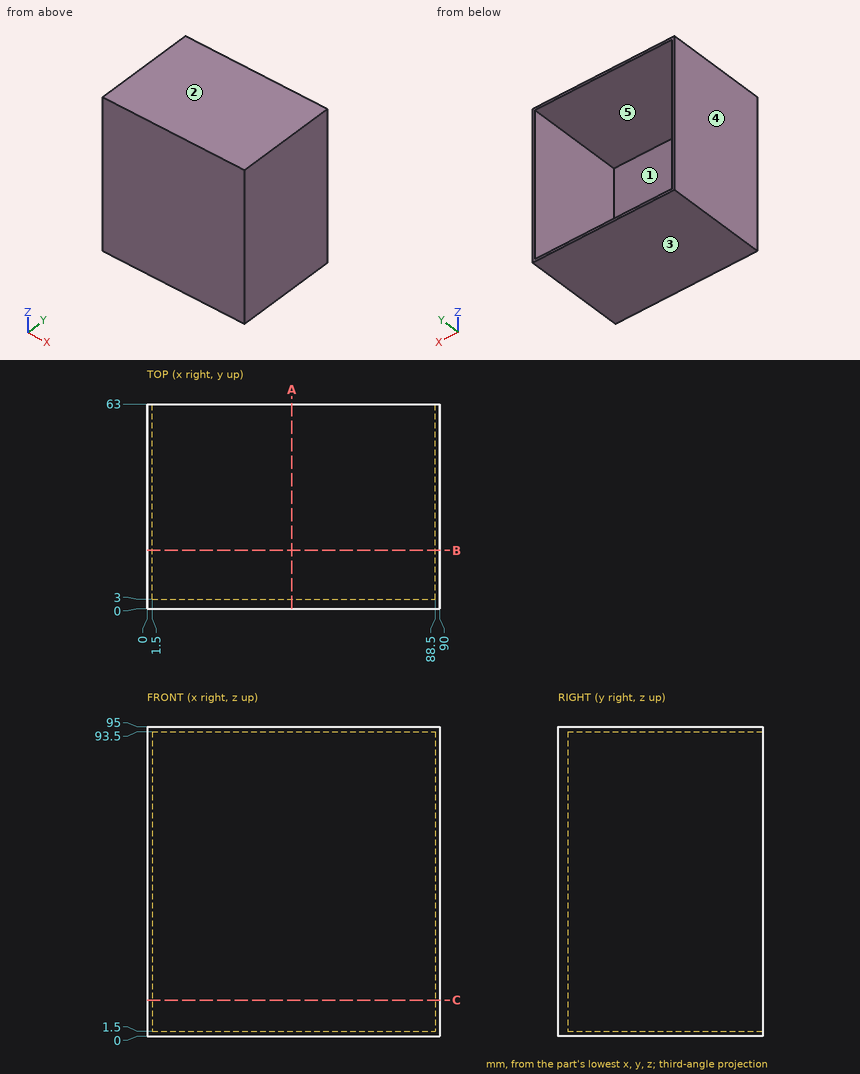
Check sheet for the drawn part. Datum: minimum x, y, z corner. Units: mm. A direction names the side the tool comes from. Round coordinates to 2 decimals unless told otherwise and drop trailing zeros. Write each loop counter-clockwise with the first axis right and the second up, starting at its lowest first coordinate (ties: lowest second). Pieces come first, ordered by that corner, then holes. Notation, with made-up numbers: (-25, 27.25) -> (-16, 27.25) arc R35 cw to (-16, 59.25) -> close; hole circle Ø5 at (-6.5, 48.25). An arc over 180 degrees is marked (long way). Put each result on its own line as item: value.
(1) Sectioned sample at B-B (y = 18). Enter the section's corners in (x, z).
Values found:
outline: (0, 0) -> (90, 0) -> (90, 95) -> (0, 95) -> close; hole (1.5, 1.5) -> (88.5, 1.5) -> (88.5, 93.5) -> (1.5, 93.5) -> close
(2) Mould release check, pull along Z, two halves, no side actions. Record for the marked faces 1, 2 and 3: released by +Z, released by -Z, zero draft, split by the parting line, or undercut.
Values found:
face 1: undercut
face 2: released by +Z
face 3: released by -Z
(3) Sectioned sample at C-C (z = 11). Enter the section's corners in (x, y), plus the area to 3 significant figures.
Values found:
outline: (0, 0) -> (90, 0) -> (90, 63) -> (88.5, 63) -> (88.5, 3) -> (1.5, 3) -> (1.5, 63) -> (0, 63) -> close
area: 450 mm^2
(4) Tool access check on the marked faces 4 and 5. Record the directions out of +Z, -Z, +X, -X, +Y, -Y that give a thin tool (end or side, any length) a straight path to the whole face; none if there is none.
Values found:
face 4: +Z, -Z, -X, +Y, -Y
face 5: +Y
(5) Go/stop test with a flat-tipped pin: pin 1 Ø2 at (x, z) = (60, 64) entering from +Y. Record where the tip stops, or that it passes through.
Values found:
pin 1: stops at y = 3
(6) Material ranges on line 1 (Z direction, x = 19, y = 26.5); line 2 (X direction, y = 10, z = 83); line 3 (Y direction, x = 47, z = 8), recorded low to high.
Values found:
line 1: z = 0 to 1.5, 93.5 to 95
line 2: x = 0 to 1.5, 88.5 to 90
line 3: y = 0 to 3
(7) Sectioned sample at A-A (x = 44.5). Enter the section's corners in (y, z).
Values found:
outline: (0, 0) -> (63, 0) -> (63, 1.5) -> (3, 1.5) -> (3, 93.5) -> (63, 93.5) -> (63, 95) -> (0, 95) -> close
